The model under review builds one solid part; all positions refer to its coordinate system, in mm. Round coordinates to 2 decimals unless told otherwise and drop trailing zeros. Write each loop counter-clockwise with the first axis right and the second up, starting at its lowest first coordinate (ties: lowest second). Pieces come first, ordered by that corner, then holes. Notation, with made-up numbers: (67.25, 29.25) -> (106.25, 29.25) arc R19 cw to (106.25, 63.25) -> close; hole circle Ø7 at (49.25, 22). An arc over 180 degrees is marked (long way). Use CSV: the item, a comma, the result in double quotes. Start each with the question number.
1) Take a section at A-A, the plane x = 5. Give the boundary of the cut face in (y, z).
2) Wall thickness on probe 1 along Z at (x, y) = (6, 5); probe 2 along Y at (x, z) = (5, 7.75); probe 3 along Y at (x, z) = (8.5, 5.25): over which ranges is each line inside the solid? List them lowest first. Write a range as [from, to].
3) Take a section at B-B, the plane z = 5. Give the boundary of the cut face in (x, y), then the cut area to 3 significant figures.
4) For pin 1 Ø3 at (x, y) = (1, 166) entering from -Z, flat-tipped, find the tip position at first contact; note if it passes through.
Autodesk Inventor part; units mm, degrees
ref_plane "YZ Plane" through (0, 0, 0) normal (1, 0, 0) x (0, 1, 0)
ref_plane "XZ Plane" through (0, 0, 0) normal (0, 1, 0) x (-1, 0, 0)
ref_plane "XY Plane" through (0, 0, 0) normal (0, 0, 1) x (1, 0, 0)
sketch "スケッチ1" plane through (0, 0, 0) normal (0, 0, 1) x (1, 0, 0)
  line L0 (0, 0) -> (10, 0)
  line L1 (10, 0) -> (10, 250)
  line L2 (10, 250) -> (0, 250)
  line L3 (0, 250) -> (0, 0)
  dimension "d0" = 10
  dimension "d1" = 250
extrude "押し出し1" add sketch "スケッチ1" along normal blind 10
sketch "スケッチ2" plane through (10, 0, 0) normal (1, 0, 0) x (0, 0, -1)
  line L0 (0, 0) -> (-10, 0)
  line L1 (0, 250) -> (-10, 250)
  point P0 (-5, 5)
  point P1 (-5, 245)
  point P2 (-5, 0)
  point P3 (-5, 0)
  point P4 (-5, 0)
  point P5 (-5, 250)
  dimension "d4" = 5
  dimension "d5" = 5
hole "穴1" at (10, 5, 5) at (10, 245, 5) direction (-1, 0, 0) diameter 3.1 end through all
sketch "スケッチ3" plane through (0, 0, 10) normal (0, 0, 1) x (1, 0, 0)
  line L0 (0, 0) -> (10, 0)
  point P0 (5, 17.5)
  point P1 (5, 0)
  point P2 (5, 0)
  dimension "d13" = 17.5
hole "穴2" at (5, 17.5, 10) direction (0, 0, -1) diameter 3.1 end through all
properties part number "Tate"
Values found:
1,outline,"(0, 0) -> (15.95, 0) -> (15.95, 10) -> (0, 10) -> close; (19.05, 0) -> (250, 0) -> (250, 10) -> (19.05, 10) -> close; hole circle Ø3.1 at (5, 5); hole circle Ø3.1 at (245, 5)"
2,probe 1,"[0, 3.45], [6.55, 10]"
2,probe 2,"[0, 15.95], [19.05, 250]"
2,probe 3,"[0, 3.47], [6.53, 243.47], [246.53, 250]"
3,outline,"(0, 0) -> (10, 0) -> (10, 3.45) -> (0, 3.45) -> close; (0, 6.55) -> (10, 6.55) -> (10, 243.45) -> (0, 243.45) -> close; (0, 246.55) -> (10, 246.55) -> (10, 250) -> (0, 250) -> close; hole circle Ø3.1 at (5, 17.5)"
3,area,"2,430 mm²"
4,pin 1,"z = 0"
